from build123d import *

# Parameters (mm, degrees)
BOSS_EXTRUDE1_DEPTH     = 1026
CUT_EXTRUDE1_DEPTH      = 9844.379832938
CUT_EXTRUDE1_DEPTH_BACK = 9844.379832938
SKETCH2_R               = 11


with BuildPart() as part:
    # Sketch1 → Boss-Extrude1 (new body)
    with BuildSketch(Plane.XY):
        Polygon((-11592.288440525, 7313.590405803), (-11721.096751517, 7351.933229733), (-11720.288440525, 7356.867460508), (-11592.288440525, 7318.657051678), (-11425.788440525, 7356.867460508), (-11395.788440525, 7356.867460508), (-11395.788440525, 7351.867460508), (-11425.381609332, 7351.867460508), align=None)
    extrude(amount=BOSS_EXTRUDE1_DEPTH)

    # Sketch2 → Cut-Extrude1 (cut, two sides: drawn at the far end of the back side and taken through both)
    with BuildSketch(Plane(origin=(-2172.647475249, 9473.814226158, 0), x_dir=(0.9746972479016649, 0.22352913665318996, 0), z_dir=(0.22352913665318996, -0.9746972479016649, 0)).offset(-CUT_EXTRUDE1_DEPTH_BACK)):
        with Locations(Location((-9664.171090618, 50, 0), (0, 0, 275.90955698))):
            Circle(SKETCH2_R)
        with Locations(Location((-9664.171090618, 150, 0), (0, 0, 275.90955698))):
            Circle(SKETCH2_R)
        with Locations(Location((-9664.171090618, 392, 0), (0, 0, 275.90955698))):
            Circle(SKETCH2_R)
        with Locations(Location((-9664.171090618, 876, 0), (0, 0, 275.90955698))):
            Circle(SKETCH2_R)
        with Locations(Location((-9664.171090618, 976, 0), (0, 0, 275.90955698))):
            Circle(SKETCH2_R)
        with Locations(Location((-9664.171090618, 634, 0), (0, 0, 275.90955698))):
            Circle(SKETCH2_R)
    extrude(amount=CUT_EXTRUDE1_DEPTH + CUT_EXTRUDE1_DEPTH_BACK, mode=Mode.SUBTRACT)


solid = part.part
Verification items for the finished model (mm, model axes). A direction names the side the tool comes from. Coordinates: 2 decimals unless noted, no trailing zeros. Write each loop counter-clockwise with the first axis right and the second up, starting at its lowest first coordinate (ties: lowest second). Pieces come first, ordered by that corner, then holes. Notation, with made-up numbers: M 4.25,2 L 24.25,2 A27 cw 24.25,29 Z; hole C 84,17.25 d9. An arc over 180 degrees is marked long. Use a Markdown table: item, result.
Q1. Draft check along Z on faces 3 (the face through (-11596.404, 7317.47, 139.459)), 4 (the face through (-11410, 7351.867, 506)), 5 (the face through (-11558, 7326, 0)). Enter one of: +Z half, -Z half, draft (parallel to the pull), parting line (faces both ways), or undercut.
Reply:
| item | result |
|---|---|
| face 3 | undercut |
| face 4 | draft |
| face 5 | -Z half |
Q2. Set-up check for faces 1 (the face through (-11657.18, 7338.03, 505.82)), 2 (the face through (-11655.791, 7332.493, 505.818)): record each of +Z, -Z, +X, -X, +Y, -Y from which the full face is reachable in a straight line by a thin tool's end or side.
Reply:
| item | result |
|---|---|
| face 1 | +Z, -Z, +Y |
| face 2 | +Z, -Z, -X, -Y |
Q3. Sectioned sample at D-D, the plane x = -11624. Record the boundary of the cut face in (y, z).
Reply:
| item | result |
|---|---|
| outline | M 7323.03,0 L 7328.12,0 L 7328.12,1026 L 7323.03,1026 Z |
Q4. Thickness scan on line 1 (Y direction, x = -11443, z = 377); line 2 (Y direction, x = -11480, z = 327). Record the ranges inside material, lowest first.
Reply:
| item | result |
|---|---|
| line 1 | y = 7347.83 to 7352.92 |
| line 2 | y = 7339.34 to 7344.43 |
Q5. Sectioned sample at C-C, the plane x = -11675. Record the boundary of the cut face in (y, z).
Reply:
| item | result |
|---|---|
| outline | M 7338.21,0 L 7343.35,0 L 7343.35,1026 L 7338.21,1026 Z |
Q6. Sectioned sample at B-B, the plane z = 749.5. Record the boundary of the cut face in (x, y), plus the area to 3 significant figures.
Reply:
| item | result |
|---|---|
| outline | M -11721.1,7351.93 L -11592.29,7313.59 L -11425.38,7351.87 L -11395.79,7351.87 L -11395.79,7356.87 L -11425.79,7356.87 L -11592.29,7318.66 L -11720.29,7356.87 Z |
| area | 1,650 mm² |
Q7. Go/stop test with flat-tipped pins: P1, Ø5, axis at x = -11658, z = 117.5, coming from the -Y side; P2, Ø23.5, axis at x = -11410, z = 659, coming from the -Y side. Record where each tip stops, or that it passes through.
Reply:
| item | result |
|---|---|
| P1 | stops at y = 7332.41 |
| P2 | stops at y = 7351.87 |
Q8. Sectioned sample at A-A, the plane y = 7331. Record the boundary of the cut face in (x, z).
Reply:
| item | result |
|---|---|
| outline | M -11650.77,0 L -11633.64,0 L -11633.64,1026 L -11650.77,1026 Z; M -11538.5,0 L -11516.37,0 L -11516.37,1026 L -11538.5,1026 Z |
